Autodesk Fusion 360 part; units mm, degrees
sketch "スケッチ1" plane through (0, 0, 0) normal (0, 1, 0) x (1, 0, 0)
  circle A0 centre (0, 0) radius 14.8
  curve L0
  dimension "d1" = 29.6
extrude "押し出し1" add sketch "スケッチ1" along normal blind 10 makes body 1
sketch "スケッチ2" plane through (0, 10, 0) normal (0, 1, 0) x (-1, 0, 0)
  circle A0 centre (0, 0) radius 14.8
  circle A1 centre (0, 0) radius 16.5
  line L0 (1.8, 16.1642) -> (-1.8, 16.1642)
  line L1 (-2, 15.9642) -> (-2, 14.6642)
  line L2 (-2, 14.6642) -> (2, 14.6642)
  line L3 (2, 14.6642) -> (2, 15.9642)
  circle A2 centre (0, 0) radius 14.8
  arc A3 (-1.8, 16.1642) -> (-2, 15.9642) centre (-1.8, 15.9642) ccw
  arc A4 (2, 15.9642) -> (1.8, 16.1642) centre (1.8, 15.9642) ccw
  curve L4
  point P0 (2, 16.1642)
  point P1 (-2, 16.1642)
  dimension "d4" = 33
  dimension "d38" = 4
  dimension "d39" = 1.5
  dimension "d40" = 0.2
  dimension "d41" = 0.2
extrude "押し出し2" add sketch "スケッチ2" along normal blind 19 contours A0 L2 A2 | A0 L2 A2 | A0 L0 L1 L3 A2 A3 A4 | A1 bodies 1
ref_plane "作業平面1" through (0, 24, 0) normal (0, 1, 0) x (-1, 0, 0)
sketch "スケッチ3" plane through (0, 24, 0) normal (0, 1, 0) x (1, 0, 0)
ref_plane "作業平面2" through (0, 29, 0) normal (0, -1, 0) x (-1, 0, 0)
sketch "スケッチ8" plane through (0, 0, 0) normal (0, 0, 1) x (1, 0, 0)
  line L0 (0, 28.5387) -> (19, 28.5387)
  line L1 (19, 28.5387) -> (19, 29)
  line L2 (19, 29) -> (14, 30.9887)
  line L3 (14, 30.9887) -> (0, 30.9887)
  line L4 (0, 30.9887) -> (0, 28.5387)
  curve L5
  line L6 (0, 1.75) -> (0, 22.5)
  dimension "d26" = 2.45
  dimension "d30" = 14
revolve "回転1" add sketch "スケッチ8" angle 360 about axis through (0, 30.9887, 0) along (0, -1, 0) bodies 1
ref_plane "作業平面9" through (0, 31.5387, 0) normal (0, -1, 0) x (0, 0, -1)
sketch "スケッチ11" plane through (0, 31.5387, 0) normal (0, -1, 0) x (1, 0, 0)
  circle A0 centre (0, 0) radius 14
  dimension "d29" = 28
extrude "押し出し6" add sketch "スケッチ11" along normal blind 1 bodies 1
sketch "スケッチ16" plane through (0, 29, 0) normal (0, -1, 0) x (1, 0, 0)
  line L0 (-1.4356, 18.4) -> (1.5644, 18.4)
  line L1 (1.5644, 18.4) -> (1.5644, 15.4)
  line L2 (1.5644, 15.4) -> (-1.4356, 15.4)
  line L3 (-1.4356, 15.4) -> (-1.4356, 18.4)
  curve L4
  dimension "d48" = 3
  dimension "d49" = 18.4
  dimension "d50" = 3
extrude "押し出し8" add sketch "スケッチ16" along normal blind 2 bodies 1
sketch "スケッチ19" plane through (0, 0, 0) normal (0, 1, 0) x (1, 0, 0)
  circle A0 centre (0, 0) radius 13.5
  dimension "d53" = 27
extrude "押し出し9" cut sketch "スケッチ19" along normal blind 26 bodies 1
sketch "スケッチ20" plane through (0, 0, 0) normal (0, 1, 0) x (1, 0, 0)
  line L0 (-5, -15) -> (5, -15)
  line L1 (5, -15) -> (5, -12)
  line L2 (5, -12) -> (-5, -12)
  line L3 (-5, -12) -> (-5, -15)
  line L4 (0, -1.75) -> (0, -22.5)
  dimension "d56" = 10
  dimension "d58" = 3
  dimension "d59" = 15
extrude "押し出し10" cut sketch "スケッチ20" along normal blind 6 bodies 1
copy_body "ボディ -> コンポーネント1" bodies 1 removing the originals makes body 2 in component "btn"
thread "ねじ1" in component "btn"
component "btn" placed x (1, 0, 0) y (0, 1, 0) z (0, 0, 1) at (0, 0, 0)
Can you work these out from the model? Positions are in its coordinate system, mm. A direction names the side the tool comes from. Round coordinates to 2 decimals unless told otherwise and drop trailing zeros. Loops run counter-clockwise (first coordinate to the right, second up) from the corner with the lowest first, then second, coordinate; pieces in that order, holes last. Notation, with made-up numbers: (-7.5, -24) - (36.5, -24) arc R23 cw to (36.5, -6) - close; hole circle Ø6 at (52.25, -14). An arc over 180 degrees is marked (long way). Answer in a Markdown table with one row per item. Add a question column.
Q1. For pin 1 Ø0.8 at (y, z) = (28, 17) entering from +X; pin 2 Ø10 at (x, z) = (1.5, 0) entering from -Y; pin 3 Ø6 at (y, z) = (4, -8) entering from +X, each with a flat end and sliding along its axis, tell me the tip position at first contact or that it passes through.
Q2. Which directions (+Z, -Z, +X, -X, +Y, -Y) give clear straight access to the entire face, cutting with the end or side of a thin tool? Please do faces 5 (the cylindrical face through (12.932, 31.268, 5.362)), 6 (the flat face through (5, 3, 13)), 7 (the cylindrical face through (-15.24, 19.14, 6.32)), 8 (the flat face through (1.564, 28, 17)), 9 (the cylindrical face through (8.767, 28.773, 16.856)).
Q3. We'd pull the mould along X, two halves only. Please class faces 1 (the flat face through (0, 6, 14)), 2 (the flat face through (-1.436, 28, 17)), 3 (the flat face through (0, 28, 18.4)), 4 (the cylindrical face through (-2.93, 12.82, -13.18)): pulls with the +X half, pulls with the -X half, needs draft (parallel to the pull), parting line crosses it, or undercut.
Q4. I need wall thicknesses on L1, parallel to Z at x = 0, y = 8; L2, parallel to Z at x = 0, y = 12. Which ranges of each line are inside material? Lowest first, please.
Q5. I want a section at C-C on y = 13.5. List the corners of the cut face in (x, z) for me.
Q6. I want a section at B-B on z = 0. List the corners of the cut face in (x, y) for me.
Q7. I want a section at A-A on x = 0. List the corners of the cut face in (y, z) for me, and give its area (3 significant figures).
A:
| question | item | result |
|---|---|---|
| 1 | pin 1 | x = 1.56 |
| 1 | pin 2 | y = 26 |
| 1 | pin 3 | x = 13.93 |
| 2 | face 5 | +Y |
| 2 | face 6 | +Z, -Y |
| 2 | face 7 | -Y |
| 2 | face 8 | +Z, +X, -Y |
| 2 | face 9 | +Y, -Y |
| 3 | face 1 | undercut |
| 3 | face 2 | pulls with the -X half |
| 3 | face 3 | needs draft |
| 3 | face 4 | undercut |
| 4 | L1 | -14.8 to -13.5, 13.5 to 14.8 |
| 4 | L2 | -16.5 to -13.5, 13.5 to 16.5 |
| 5 | outline | circle Ø33 at (0, 0); hole circle Ø27 at (0, 0) |
| 6 | outline | (-19, 28.54) - (-16.5, 28.54) - (-16.5, 10) - (-14.8, 10) - (-14.8, 0) - (-13.5, 0) - (-13.5, 26) - (13.5, 26) - (13.5, 0) - (14.8, 0) - (14.8, 10) - (16.5, 10) - (16.5, 28.54) - (19, 28.54) - (19, 29) - (14, 30.99) - (14, 31.54) - (-14, 31.54) - (-14, 30.99) - (-19, 29) - close |
| 7 | outline | (0, -14.8) - (10, -14.8) - (10, -16.5) - (28.54, -16.5) - (28.54, -19) - (29, -19) - (30.99, -14) - (31.54, -14) - (31.54, 14) - (30.99, 14) - (29, 19) - (28.54, 19) - (28.54, 18.4) - (27, 18.4) - (27, 16.5) - (10, 16.5) - (10, 14.8) - (6, 14.8) - (6, 13.5) - (26, 13.5) - (26, -13.5) - (0, -13.5) - close |
| 7 | area | 299 mm^2 |
